Geometry check sheet. Reference: the model listing, model coordinates, mm. Give positions to 0.01 mm unless a question says otherwise; leave off trailing zeros. Loops run counter-clockwise (first coordinate to the right, second up) from the corner with the lowest first, then second, coordinate; pieces in that order, holes last. Notation, with made-up numbers: (18.25, 52) -> (39.25, 52) arc R9 cw to (39.25, 66) -> close; hole circle Ø9 at (-26.75, 1.25). An arc over 180 degrees is marked (long way). One line per question, with ' | ' between items.
Autodesk Inventor part; units mm, degrees
ref_plane "YZ Plane" through (0, 0, 0) normal (1, 0, 0) x (0, 1, 0)
ref_plane "XZ Plane" through (0, 0, 0) normal (0, 1, 0) x (-1, 0, 0)
ref_plane "XY Plane" through (0, 0, 0) normal (0, 0, 1) x (1, 0, 0)
sketch "Skizze1" plane through (0, 0, 0) normal (0, 0, 1) x (1, 0, 0)
  line L0 (-88.6, 55.38) -> (88.6, 55.38)
  line L1 (96.48, 47.5) -> (96.48, -47.5)
  line L2 (88.6, -55.38) -> (-88.6, -55.38)
  line L3 (-96.48, -47.5) -> (-96.48, 47.5)
  arc A0 (-88.6, 55.38) -> (-96.48, 47.5) centre (-88.6, 47.5) ccw
  arc A1 (-96.48, -47.5) -> (-88.6, -55.38) centre (-88.6, -47.5) ccw
  arc A2 (88.6, -55.38) -> (96.48, -47.5) centre (88.6, -47.5) ccw
  arc A3 (96.48, 47.5) -> (88.6, 55.38) centre (88.6, 47.5) ccw
  point P0 (0, 0)
  point P1 (96.48, -55.38)
  point P2 (96.48, 55.38)
  point P3 (-96.48, -55.38)
  point P4 (96.48, 0)
  point P5 (0, -55.38)
  dimension "d0" = 192.96
  dimension "d1" = 110.76
  dimension "d2" = 7.88
extrude "Extrusion1" add sketch "Skizze1" against normal blind 0.7
sketch "Skizze2" plane through (0, 0, 0) normal (0, 0, 1) x (1, 0, 0)
  line L0 (-77.44, 43.36) -> (77.44, 43.36)
  line L1 (77.44, 43.36) -> (77.44, -43.36)
  line L2 (77.44, -43.36) -> (-77.44, -43.36)
  line L3 (-77.44, -43.36) -> (-77.44, 43.36)
  point P0 (0, 0)
  point P1 (77.44, 0)
  point P2 (0, 43.36)
  dimension "d5" = 154.88
  dimension "d6" = 86.72
extrude "Extrusion2" cut sketch "Skizze2" against normal up to surface (0.7 mm away)
properties part number "Display Lens"
Item 1: Scan lines: probe 1 along Y at (x, z) = (26, -0.4); probe 2 along X at (y, z) = (-1, -0.5); probe 3 along X at (y, z) = (-51, -0.15). Record each from-to range of solid material in increasing order.
Result:
probe 1: -55.38 to -43.36, 43.36 to 55.38 | probe 2: -96.48 to -77.44, 77.44 to 96.48 | probe 3: -95.66 to 95.66
Item 2: Sectioned sample at B-B (z = -0.4). Record the cut outline in (x, y), plus the area to 3 significant figures.
Result:
outline: (-96.48, -47.5) arc R7.88 ccw to (-88.6, -55.38) -> (88.6, -55.38) arc R7.88 ccw to (96.48, -47.5) -> (96.48, 47.5) arc R7.88 ccw to (88.6, 55.38) -> (-88.6, 55.38) arc R7.88 ccw to (-96.48, 47.5) -> close; hole (-77.44, -43.36) -> (77.44, -43.36) -> (77.44, 43.36) -> (-77.44, 43.36) -> close | area: 7,890 mm2
Item 3: Sectioned sample at A-A (y = -6). Record the cut outline in (x, z).
Result:
outline: (-96.48, -0.7) -> (-77.44, -0.7) -> (-77.44, 0) -> (-96.48, 0) -> close; (77.44, -0.7) -> (96.48, -0.7) -> (96.48, 0) -> (77.44, 0) -> close
Item 4: Sectioned sample at C-C (x = 49). Record the cut outline in (y, z).
Result:
outline: (-55.38, -0.7) -> (-43.36, -0.7) -> (-43.36, 0) -> (-55.38, 0) -> close; (43.36, -0.7) -> (55.38, -0.7) -> (55.38, 0) -> (43.36, 0) -> close
